Job drawing, mm, ordinate dimensions from the low corner. One solid piece. A direction names the side the tool comes from. Give positions to 0.01 mm unless a question says otherwise; leave off trailing zeros. Order: outer loops, then holes, each group sorted by start corner. A loop starts at its lowest first (then second) coordinate and runs counter-clockwise, first axis right, second up. Notation, with made-up numbers: M 80,80 L 139,80 A22 cw 139,98 Z; hole C 31,38.25 d2. An arc over 180 degrees is marked long. Put each result on its own line as item: value. Start each with the question number.
1) Cut at A-A (y = 15). Write the cut outline in (x, z), and give its area (3 significant figures).
2) Cut at C-C (y = 7). Write the cut outline in (x, z).
3) Tool access for the marked faces 1 and 2: list every direction of +Z, -Z, +X, -X, +Y, -Y with a clear straight run to the whole face (end or side of a thin tool).
4) Drill centre lines: line 1 (X direction, y = 5, z = 5); line 2 (Y direction, x = 4.5, z = 24); line 3 (X direction, y = 15.75, z = 5). Where is each one in solid material? Low to high. Write a range as [from, to].
5) Cut at B-B (z = 5). Write the cut outline in (x, y).
6) Two-plate mould, pull along Z, no slides. Class the marked faces 3, 4 and 5: released by +Z, released by -Z, zero draft, split by the parting line, or undercut.
7) Pin check, flat tips, straight feed: pin 1 (4 mm diameter, centred on x = 18, z = 22.5, fed in from -Y); pin 2 (2 mm diameter, centred on x = 12, z = 29, fed in from -Y). Stop position of each tip, or through.
8) Cut at D-D (x = 12.5). Write the cut outline in (y, z).
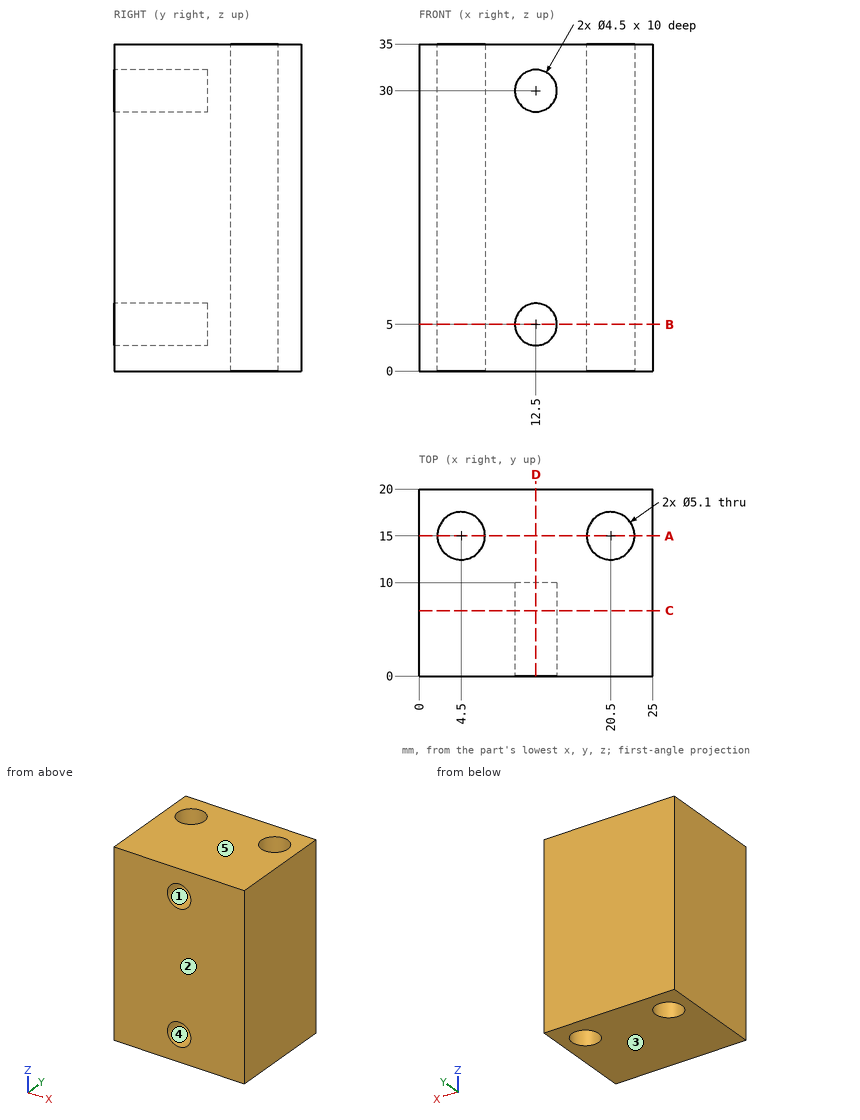
Solution:
1. outline: M 0,0 L 1.95,0 L 1.95,35 L 0,35 Z; M 7.05,0 L 17.95,0 L 17.95,35 L 7.05,35 Z; M 23.05,0 L 25,0 L 25,35 L 23.05,35 Z
1. area: 518 mm²
2. outline: M 0,0 L 25,0 L 25,35 L 0,35 Z; hole C 12.5,5 d4.5; hole C 12.5,30 d4.5
3. face 1: -Y
3. face 2: +Z, -Z, +X, -X, -Y
4. line 1: [0, 10.25], [14.75, 25]
4. line 2: [0, 12.45], [17.55, 20]
4. line 3: [0, 2.06], [6.94, 18.06], [22.94, 25]
5. outline: M 0,0 L 10.25,0 L 10.25,10 L 14.75,10 L 14.75,0 L 25,0 L 25,20 L 0,20 Z; hole C 4.5,15 d5.1; hole C 20.5,15 d5.1
6. face 3: released by -Z
6. face 4: undercut
6. face 5: released by +Z
7. pin 1: y = 0
7. pin 2: y = 10
8. outline: M 0,0 L 20,0 L 20,35 L 0,35 L 0,32.25 L 10,32.25 L 10,27.75 L 0,27.75 L 0,7.25 L 10,7.25 L 10,2.75 L 0,2.75 Z
